The model under review builds one solid part; all positions refer to its coordinate system, in mm. A direction names the side the tool comes from. Round coordinates to 2 decimals unless told otherwise and drop trailing zeros. Order: outer loops, then holes, each group sorted by start corner. A loop starts at its lowest first (then second) coordinate and runs counter-clockwise, first axis right, second up.
Autodesk Inventor part; units mm, degrees
ref_plane "Work Plane2" through (0, 0, -19.05) normal (0, 0, 1) x (1, 0, 0)
ref_plane "YZ Plane" through (0, 0, 0) normal (1, 0, 0) x (0, 1, 0)
ref_plane "XZ Plane" through (0, 0, 0) normal (0, 1, 0) x (-1, 0, 0)
sketch "Sketch9" plane through (0, 0, 0) normal (0, 1, 0) x (-1, 0, 0)
  circle A0 centre (0, 0) radius 19.05
  dimension "d53" = 38.1
extrude "Extrusion6" add sketch "Sketch9" along normal mid plane 27.432
sketch "Sketch10" plane through (0, 13.716, 0) normal (0, 1, 0) x (1, 0, 0)
  circle A0 centre (0, 0) radius 13.589
  dimension "idWasher" = 27.178
extrude "Extrusion7" add sketch "Sketch10" along normal blind 3.556
sketch "Sketch11" plane through (0, 17.272, 0) normal (0, 1, 0) x (1, 0, 0)
  line L0 (7.6623, 0) -> (3.8312, -6.6358)
  line L1 (3.8312, -6.6358) -> (-3.8312, -6.6358)
  line L2 (-3.8312, -6.6358) -> (-7.6623, 0)
  line L3 (-7.6623, 0) -> (-3.8312, 6.6357)
  line L4 (-3.8312, 6.6357) -> (3.8312, 6.6357)
  line L5 (3.8312, 6.6357) -> (7.6623, 0)
  point P0 (0, 0)
  point P1 (0, 0)
  dimension "d59" = 13.2715
extrude "Extrusion8" cut sketch "Sketch11" against normal through all
sketch "Sketch12" plane through (0, 0, 0) normal (1, 0, 0) x (0, 1, 0)
  circle A0 centre (-4.572, 9.1758) radius 2.54
  line L0 (17.272, 0) -> (-13.716, 0)
  line L1 (-13.716, 19.05) -> (-13.716, -19.05)
  point P0 (0, 0)
  dimension "d62" = 5.08
  dimension "d63" = 9.1758
  dimension "oneThirdSpoolHeight" = 9.144
extrude "Extrusion9" cut sketch "Sketch12" along normal through all both and the other way through all
chamfer "Chamfer5" distance 3.175 angle 45 2 edges at (16.6229, -7.1087, 9.3048) (-16.6229, -7.1087, 9.3048)
ref_plane "Work Plane2" through (0, 0, -19.05) normal (0, 0, 1) x (1, 0, 0)
sketch "Sketch13" plane through (0, 0, -19.05) normal (0, 0, 1) x (1, 0, 0)
  point P0 (0, 0)
  point P1 (0, 0)
hole "Hole2" at (0, 0, -19.05) direction (0, 0, 1) diameter 4.699 depth 12.4143 counterbore diameter 5.5372 counterbore depth 5.5626
chamfer "Chamfer6" distance 1.5875 angle 45 12 edges at (-5.7467, 17.272, -3.3179) (0, 17.272, -6.6357) (5.7467, 17.272, -3.3179) (5.7467, 17.272, 3.3179) (0, 17.272, 6.6358) (-5.7467, 17.272, 3.3179) (0, -13.716, 6.6358) (5.7467, -13.716, 3.3179) (5.7467, -13.716, -3.3179) (0, -13.716, -6.6357) (-5.7467, -13.716, -3.3179) (-5.7467, -13.716, 3.3179)
equation "\"d53\" = spoolInteriorDiameter"
equation "\"d59\" = hexDiameter"
equation "\"d62\" = holeForString"
equation "\"d63\" = stringHoleCenterFromHexShaft"
equation "\"oneThirdSpoolHeight\" = 0.333333 * singleSpoolHeight"
equation "\"d67\" = stringHoleChamfer"
equation "\"d77\" = hexHoleChamfer"
equation "\"holeForString\" = stringDiameter + clearanceForString"
equation "\"stringDiameter\" = 3.048"
equation "\"clearanceForString\" = 2.032"
equation "\"spoolHeightWithoutSpacer\" = 69.85"
equation "\"hexShaftDiameter\" = 12.7"
equation "\"clearanceForHexShaft\" = 0.5715"
equation "\"hexDiameter\" = hexShaftDiameter + clearanceForHexShaft"
equation "\"supportChannels\" = 3.81"
equation "\"spoolInteriorDiameter\" = 38.1"
equation "\"spoolInteriroRadius\" = 0.5 * spoolInteriorDiameter"
equation "\"spoolExteriorDiameter\" = 88.9"
equation "\"spoolExteriorRadius\" = 0.5 * spoolExteriorDiameter"
equation "\"spoolFiletRadius\" = 0.5 * supportChannels"
equation "\"holeCenter\" = 0.25 * spoolHeightWithoutSpacer - 0.75 * supportChannels"
equation "\"hexHoleChamfer\" = 1.5875"
equation "\"stringHoleCenterFromHexShaft\" = 0.5 * hexDiameter + 0.5 * holeForString"
equation "\"textCircleDiameter\" = 0.75 * spoolExteriorDiameter"
equation "\"textHeight\" = 6.096"
equation "\"textDepth\" = 1.27"
equation "\"stringHoleChamfer\" = 3.175"
equation "\"spoolTotalHeight\" = 76.2"
equation "\"spaceHeight\" = spoolTotalHeight - spoolHeightWithoutSpacer"
equation "\"spacerDiameter\" = 24.13"
properties part number "2SidedSpoolV04" material "PC/ABS Plastic"
(1) Consider section D-D (z = -12). Write out the cut boundary in (x, y), and give its area (3 significant figures).
Data:
outline: (-14.8, -13.72) - (14.8, -13.72) - (14.8, 13.72) - (6.38, 13.72) - (6.38, 17.27) - (-6.38, 17.27) - (-6.38, 13.72) - (-14.8, 13.72) - close; hole circle Ø4.7 at (0, 0)
area: 840 mm2
(2) Consider section B-B (y = 9.5). Write out the cut boundary in (x, z), and give its area (3 significant figures).
Data:
outline: circle Ø38.1 at (0, 0); hole (-7.66, 0) - (-3.83, -6.64) - (3.83, -6.64) - (7.66, 0) - (3.83, 6.64) - (-3.83, 6.64) - close
area: 988 mm2
(3) To check wall thickness, follow probe 1 along Y at (x, z) = (-7, 9); probe 2 along Y at (x, z) = (0, -8.5); probe 3 along Z at (x, y) = (-2, -5.5). State the ranges of each line that lie inside material, in increasing order.
Data:
probe 1: y = -13.72 to -7.11, -2.04 to 17.27
probe 2: y = -13.72 to -2.35, 2.35 to 17.27
probe 3: z = -18.94 to -6.64, 6.64 to 6.81, 11.54 to 18.94
(4) For faces 1 (the flat face through (6.48, 16.49, 3.66)), 2 (the flat face through (2, 2, -6.636)), 3 (the cylindrical face through (-2.33, -0.31, -10.01)), list the 3-axis set-ups (+Z, -Z, +X, -X, +Y, -Y) from which the entire face can be reached by the end or side of a thin tool; tool diameter is ignored.
Data:
face 1: +Y
face 2: +Y, -Y
face 3: -Z
(5) Consider section A-A (x = 0). Write out the cut boundary in (y, z), and give its area (3 significant figures).
Data:
outline: (-13.72, -19.05) - (-2.77, -19.05) - (-2.77, -13.49) - (-2.35, -13.49) - (-2.35, -6.64) - (-12.13, -6.64) - (-13.72, -8.22) - close; (-13.72, 8.22) - (-12.13, 6.64) - (15.68, 6.64) - (17.27, 8.22) - (17.27, 13.59) - (13.72, 13.59) - (13.72, 19.05) - (-13.72, 19.05) - close; (2.35, -13.49) - (2.77, -13.49) - (2.77, -19.05) - (13.72, -19.05) - (13.72, -13.59) - (17.27, -13.59) - (17.27, -8.22) - (15.68, -6.64) - (2.35, -6.64) - close; hole circle Ø5.08 at (-4.57, 9.18)
area: 642 mm2
(6) Insertion check: pin 1 (1 mm diameter, centred on x = -3.5, z = -7.5, fed in from +Y); pin 2 (2 mm diameter, centred on x = -6.5, y = 3, fed in from -Z); pin 3 (5 mm diameter, centred on x = -3, y = 12, fed in from +Z). Each pin has a flat end and moves straight along its axis. Give the tip position at first contact, or say it passes through.
Data:
pin 1: stops at y = 17.05
pin 2: stops at z = -18.24
pin 3: stops at z = 19.04
(7) Draft analysis for pull direction X (two halves, no side actions). For faces 4 (the flat face through (13, 13.716, 5)), 5 (the cylindrical face through (2.48, 2.856, -18.888)), 6 (the flat face through (6.41, 16.49, -3.78)), state which applies: pulls with the +X half, pulls with the -X half, needs draft (parallel to the pull), parting line crosses it, or undercut.
Data:
face 4: needs draft
face 5: parting line crosses it
face 6: undercut
(8) Consider section C-C (z = -0.5). Write out the cut boundary in (x, y), and give its area (3 significant figures).
Data:
outline: (-19.04, -13.72) - (-9.21, -13.72) - (-7.37, -12.13) - (-7.37, 15.68) - (-9.21, 17.27) - (-13.58, 17.27) - (-13.58, 13.72) - (-19.04, 13.72) - close; (7.37, -12.13) - (9.21, -13.72) - (19.04, -13.72) - (19.04, 13.72) - (13.58, 13.72) - (13.58, 17.27) - (9.21, 17.27) - (7.37, 15.68) - close
area: 679 mm2
